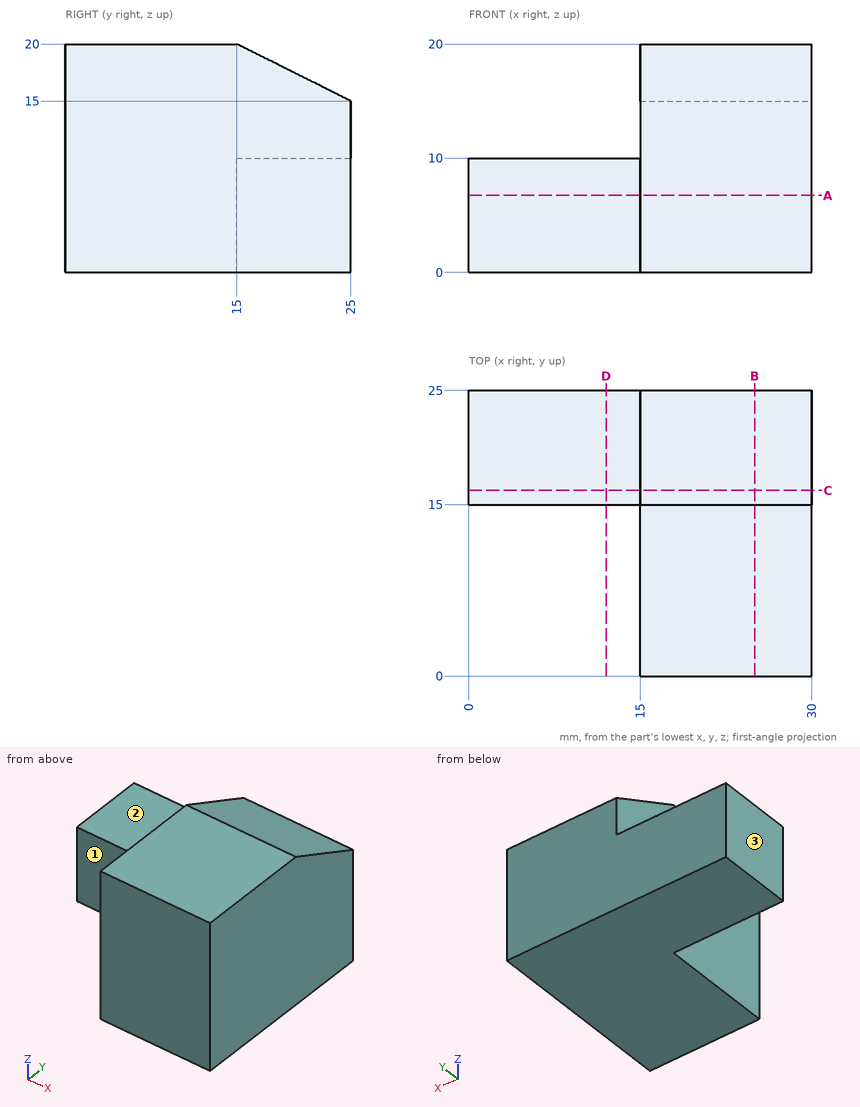
Study the drawing (mm; zero at the part's minimum x, y, z) and answer. A direction names the side the tool comes from. Give positions to 0.01 mm unless a question says otherwise; leave off trailing zeros. Order: outer loops, then holes, each group sorted by start corner. A loop starts at its lowest first (then second) coordinate and runs counter-clockwise, first axis right, second up.
1) Find section B-B on x = 25. Write down the section's boundary in (y, z), then the cut area to 3 significant figures.
Reported:
outline: (0, 0) - (25, 0) - (25, 15) - (15, 20) - (0, 20) - close
area: 475 mm2
2) Find section D-D on x = 12. Write down the section's boundary in (y, z), then the cut area to 3 significant figures.
Reported:
outline: (15, 0) - (25, 0) - (25, 10) - (15, 10) - close
area: 100 mm2
3) Find section A-A on z = 6.75. Write down the section's boundary in (x, y).
Reported:
outline: (0, 15) - (15, 15) - (15, 0) - (30, 0) - (30, 25) - (0, 25) - close
4) Consider line 1 along X through (y, z) = (14, 10.5); line 2 along Y through (x, z) = (13.5, 8.75); line 3 along Z through (x, y) = (2, 21.5). Determine where each line is inside the solid, lowest interval first.
Reported:
line 1: x = 15 to 30
line 2: y = 15 to 25
line 3: z = 0 to 10
5) Find section C-C on y = 16.25. Write down the section's boundary in (x, z) (3 decimals).
Reported:
outline: (0, 0) - (30, 0) - (30, 19.375) - (15, 19.375) - (15, 10) - (0, 10) - close
6) Given P1, Ø3, axis at x = 12.5, z = 2, coming from the -Y side; P2, Ø2, axis at x = 13, z = 16, coming from the +Y side; P3, Ø3, axis at x = 5, y = 18, coming from the +Z side; P4, Ø1.5, axis at x = 23, y = 17, coming from the +Z side (3 decimals), each flat-ended and moving along its own axis, determine where each tip first touches the part or whether it passes through.
Reported:
P1: stops at y = 15
P2: passes through
P3: stops at z = 10
P4: stops at z = 19.375
7) For the marked faces 1, 2 and 3, determine the directions among +Z, -Z, +X, -X, +Y, -Y from which every point of the face is accessible in a straight line to the end or side of a thin tool.
Reported:
face 1: +Z, -Z, -X, -Y
face 2: +Z, -X, +Y, -Y
face 3: +Z, -Z, -X, +Y, -Y
